Design review of the part built by this model. Coordinates are the model's own, in mm. A direction names the side the tool comes from. Coordinates: 2 decimals unless noted, no trailing zeros. Loops run counter-clockwise (first coordinate to the right, second up) from the corner with the lowest first, then second, coordinate; pieces in that order, holes last. Notation, with made-up numbers: M 70.25,0 L 102.25,0 A14 ccw 102.25,7 Z; hole C 35.5,10.5 d8. An arc over 180 degrees is marked long. Put each result on its own line as item: value. Start each with the question number.
(1) Take a section at A-A, the plane x = 0. Give the boundary of the cut face in (y, z) (3 decimals), then the cut area to 3 significant figures.
(2) Take a section at B-B, the plane z = 0. Give the boundary of the cut face in (x, y) (3 decimals), then the cut area to 3 significant figures.
(3) Take a section at D-D, the plane z = -10.16. Give the boundary of the cut face in (x, y) (3 decimals).
(4) Clearance check with flat-ended pins moving along their axes: pin 1 (2 mm diameter, centred on x = 0, z = 10.16, fed in from -Y); pin 2 (1.5 mm diameter, centred on y = 2, z = -2.5, fed in from -X). State where each tip first meets the part, or that it passes through.
(5) For faces 1 (the flat face through (-4.291, 1.61, 6.536)), 2 (the flat face through (3, 0, 3)), list the 3-axis set-ups (+Z, -Z, +X, -X, +Y, -Y) from which the entire face can be reached by the end or side of a thin tool; tool diameter is ignored.
(6) The part is to be moulded in two halves that separate along X. For faces 3 (the flat face through (7.2, 1.61, -7.17)), 4 (the flat face through (3, 3.175, 3)), 5 (the cylindrical face through (-1.82, 1.57, -13.85)), say which applies: +X half, -X half, draft (parallel to the pull), parting line (faces both ways), or undercut.
(7) Take a section at C-C, the plane y = 1.6. Give the boundary of the cut face in (x, z) (3 decimals), then the cut area to 3 significant figures.
(8) For probe 1 along Z at (x, y) = (0, 2.35) (3 decimals); probe 2 along Z at (x, y) = (2.75, 1.9); probe 3 along X at (y, z) = (2.05, -9), list the stretches that pass through material, from the lowest coordinate up. Write a range as [from, to].
```python
from build123d import *

# Parameters (mm, degrees)
SKETCH1_R           = 13.97
BOSS_EXTRUDE1_DEPTH = 3.175
SKETCH2_R           = 3.175
CUT_EXTRUDE1_DEPTH  = 3.175
CIRPATTERN1_COUNT   = 4
CUT_EXTRUDE2_DEPTH  = 5.08
CIRPATTERN2_COUNT   = 2


with BuildPart() as part:
    # Sketch1 → Boss-Extrude1 (new body)
    with BuildSketch(Plane(origin=(0, 0, 0), x_dir=(1, 0, 0), z_dir=(0, 1, 0))):
        Circle(SKETCH1_R)
    extrude(amount=BOSS_EXTRUDE1_DEPTH)

    # Sketch2 → Cut-Extrude1 (cut)
    with BuildSketch(Plane(origin=(0, 3.175, 0), x_dir=(1, 0, 0), z_dir=(0, 1, 0))):
        Circle(SKETCH2_R)
    extrude(amount=-CUT_EXTRUDE1_DEPTH, mode=Mode.SUBTRACT)

    # Sketch4 → #4 Clearance Hole1 (revolve, cut)
    with BuildSketch(Plane(origin=(0, 3.175, -10.16), x_dir=(0, 0, 1), z_dir=(1, 0, 0))):
        Polygon((0, 0), (0, 11.140574487), (1.63195, 10.16), (1.63195, 0), align=None)
    f_4_clearance_hole1 = revolve(axis=Axis((0, 9.525, -10.16), (0, -1, 0)), mode=Mode.SUBTRACT)

    # CirPattern1: #4 Clearance Hole1 ×4 about axis
    cirpattern1_axis = Axis((0, 0, 0), (0, 1, 0))
    for i in range(1, CIRPATTERN1_COUNT):
        add(f_4_clearance_hole1.rotate(cirpattern1_axis, i * 360 / CIRPATTERN1_COUNT), mode=Mode.SUBTRACT)

    # Sketch6 → Cut-Extrude2 (cut)
    with BuildSketch(Plane(origin=(0, 3.175, 0), x_dir=(1, 0, 0), z_dir=(0, 1, 0))):
        Polygon((4.714634464, 2.469570433), (8.306736912, 6.061672882), (6.061672882, 8.306736912), (2.469570433, 4.714634464), align=None)
    cut_extrude2 = extrude(amount=-CUT_EXTRUDE2_DEPTH, mode=Mode.SUBTRACT)

    # CirPattern2: Cut-Extrude2 ×2 about axis
    cirpattern2_axis = Axis((0, 0, 0), (0, 1, 0))
    for i in range(1, CIRPATTERN2_COUNT):
        add(cut_extrude2.rotate(cirpattern2_axis, i * 360 / CIRPATTERN2_COUNT), mode=Mode.SUBTRACT)


solid = part.part
```
Computed values:
1. outline: M 0,-13.97 L 3.175,-13.97 L 3.175,-11.792 L 0,-11.792 Z; M 0,-8.528 L 3.175,-8.528 L 3.175,-3.175 L 0,-3.175 Z; M 0,3.175 L 3.175,3.175 L 3.175,8.528 L 0,8.528 Z; M 0,11.792 L 3.175,11.792 L 3.175,13.97 L 0,13.97 Z
1. area: 47.8 mm^2
2. outline: M -13.97,0 L -11.792,0 L -11.792,3.175 L -13.97,3.175 Z; M -8.528,0 L -3.175,0 L -3.175,3.175 L -8.528,3.175 Z; M 3.175,0 L 8.528,0 L 8.528,3.175 L 3.175,3.175 Z; M 11.792,0 L 13.97,0 L 13.97,3.175 L 11.792,3.175 Z
2. area: 47.8 mm^2
3. outline: M -9.588,0 L -1.632,0 L -1.632,3.175 L -9.588,3.175 Z; M 1.632,0 L 9.588,0 L 9.588,3.175 L 1.632,3.175 Z
4. pin 1: passes through
4. pin 2: stops at x = -13.86
5. face 1: +Y, -Y
5. face 2: +Z, -Z, +X, -X, -Y
6. face 3: undercut
6. face 4: draft
6. face 5: parting line
7. outline: C 0,0 d27.94; hole C -10.16,0 d3.264; hole M -8.307,6.062 L -4.715,2.47 L -2.47,4.715 L -6.062,8.307 Z; hole C 0,0 d6.35; hole C 0,-10.16 d3.264; hole C 0,10.16 d3.264; hole M 2.47,-4.715 L 6.062,-8.307 L 8.307,-6.062 L 4.715,-2.47 Z; hole C 10.16,0 d3.264
7. area: 516 mm^2
8. probe 1: z = [-13.97, -11.792], [-8.528, -3.175], [3.175, 8.528], [11.792, 13.97]
8. probe 2: z = [-13.7, -5], [-4.43, -1.59], [1.59, 13.7]
8. probe 3: x = [-10.68, -1.15], [1.15, 10.68]
